```python
from build123d import *

# Parameters (mm, degrees)
SKETCH_1_W                       = 145
SKETCH_1_H                       = 80
EXTRUDE_1_DEPTH                  = 35
SKETCH_2_W                       = 141
SKETCH_2_H                       = 76
CUT_EXTRUDE_1_DEPTH              = 33
SKETCH_3_R                       = 3.5
EXTRUDE_2_DEPTH                  = 15
SKETCH_4_R                       = 1.5
CUT_EXTRUDE_2_DEPTH              = 15
SKETCH_5_W                       = 10
SKETCH_5_H                       = 10
SKETCH_5_W_2                     = 16
SKETCH_5_H_2                     = 21
CUT_EXTRUDE_3_DEPTH              = 15
SKETCH_6_W                       = 10
SKETCH_6_H                       = 10
CUT_EXTRUDE_4_DEPTH              = 15
SKETCH_9_R                       = 3.5
EXTRUDE_3_DEPTH                  = 33
SKETCH_10_R                      = 1.5
CUT_EXTRUDE_5_DEPTH              = 33
PATTERN_LINEAR_2_COUNT           = 2
PATTERN_LINEAR_2_PITCH           = 72
PATTERN_LINEAR_2_COUNT_DIR2      = 2
PATTERN_LINEAR_2_PITCH_DIR2      = 137
SKETCH_12_W                      = 2
SKETCH_12_H                      = 6
EXTRUDE_4_DEPTH                  = 5
SKETCH_13_R                      = 1.5
CUT_EXTRUDE_6_DEPTH              = 5
PATTERN_LINEAR_3_COUNT           = 2
PATTERN_LINEAR_3_PITCH           = 74
PATTERN_LINEAR_4_COUNT           = 2
PATTERN_LINEAR_4_PITCH           = 150
PATTERN_LINEAR_4_COPY_1_SKETCH_R = 1.5
PATTERN_LINEAR_4_COPY_1_DEPTH    = 5


with BuildPart() as part:
    # Эскиз1 → Бобышка-Вытянуть1 (new body)
    with BuildSketch(Plane.XY):
        with Locations((72.5, 40)):
            Rectangle(SKETCH_1_W, SKETCH_1_H)
    extrude(amount=EXTRUDE_1_DEPTH)

    # Эскиз2 → Вырез-Вытянуть1 (cut)
    with BuildSketch(Plane(origin=(0, 0, 0), x_dir=(-1, 0, 0), z_dir=(0, 0, -1))):
        with Locations((-72.5, 40)):
            Rectangle(SKETCH_2_W, SKETCH_2_H)
    extrude(amount=-CUT_EXTRUDE_1_DEPTH, mode=Mode.SUBTRACT)

    # Эскиз3 → Бобышка-Вытянуть2 (add)
    with BuildSketch(Plane(origin=(0, 0, 33), x_dir=(-1, 0, 0), z_dir=(0, 0, -1))):
        with Locations(Location((-109.79, 62.86, 0), (0, 0, 180))):
            Circle(SKETCH_3_R)
        with Locations(Location((-109.79, 17.14, 0), (0, 0, 180))):
            Circle(SKETCH_3_R)
        with Locations(Location((-34.79, 64.13, 0), (0, 0, 180))):
            Circle(SKETCH_3_R)
        with Locations(Location((-34.79, 15.87, 0), (0, 0, 180))):
            Circle(SKETCH_3_R)
    extrude(amount=EXTRUDE_2_DEPTH)

    # Эскиз4 → Вырез-Вытянуть2 (cut)
    with BuildSketch(Plane(origin=(0, 0, 18), x_dir=(-1, 0, 0), z_dir=(0, 0, -1))):
        with Locations((-109.79, 62.86)):
            Circle(SKETCH_4_R)
        with Locations((-34.79, 64.13)):
            Circle(SKETCH_4_R)
        with Locations((-34.79, 15.87)):
            Circle(SKETCH_4_R)
        with Locations((-109.79, 17.14)):
            Circle(SKETCH_4_R)
    extrude(amount=-CUT_EXTRUDE_2_DEPTH, mode=Mode.SUBTRACT)

    # Эскиз5 → Вырез-Вытянуть3 (cut)
    with BuildSketch(Plane.ZY):
        with Locations((13, 26)):
            Rectangle(SKETCH_5_W, SKETCH_5_H)
        with Locations((14, 51.5)):
            Rectangle(SKETCH_5_W_2, SKETCH_5_H_2)
    extrude(amount=-CUT_EXTRUDE_3_DEPTH, mode=Mode.SUBTRACT)

    # Эскиз6 → Вырез-Вытянуть4 (cut)
    with BuildSketch(Plane.ZY.offset(-143)):
        with Locations((13, 54)):
            Rectangle(SKETCH_6_W, SKETCH_6_H)
    extrude(amount=-CUT_EXTRUDE_4_DEPTH, mode=Mode.SUBTRACT)

    # Эскиз9 → Бобышка-Вытянуть3 (add)
    with BuildSketch(Plane(origin=(0, 0, 33), x_dir=(-1, 0, 0), z_dir=(0, 0, -1))):
        with Locations((-4, 76)):
            Circle(SKETCH_9_R)
    extrude_3 = extrude(amount=EXTRUDE_3_DEPTH)

    # Эскиз10 → Вырез-Вытянуть5 (cut)
    with BuildSketch(Plane(origin=(0, 0, 0), x_dir=(-1, 0, 0), z_dir=(0, 0, -1))):
        with Locations((-4, 76)):
            Circle(SKETCH_10_R)
    cut_extrude_5 = extrude(amount=-CUT_EXTRUDE_5_DEPTH, mode=Mode.SUBTRACT)

    # Линейный массив2: Бобышка-Вытянуть3, Cut-Extrude 5 2 × 2
    with Locations(*[(j * PATTERN_LINEAR_2_PITCH_DIR2, -i * PATTERN_LINEAR_2_PITCH, 0) for i in range(PATTERN_LINEAR_2_COUNT) for j in range(PATTERN_LINEAR_2_COUNT_DIR2) if (i, j) != (0, 0)]):
        add(extrude_3)
        add(cut_extrude_5, mode=Mode.SUBTRACT)

    # Эскиз12 → Бобышка-Вытянуть4 (add)
    with BuildSketch(Plane(origin=(145, 0, 0), x_dir=(0, 0, -1), z_dir=(1, 0, 0))):
        with Locations((-34, 77)):
            Rectangle(SKETCH_12_W, SKETCH_12_H)
        with Locations((-34, 3)):
            Rectangle(SKETCH_12_W, SKETCH_12_H)
    extrude_4 = extrude(amount=EXTRUDE_4_DEPTH)

    # Эскиз13 → Вырез-Вытянуть6 (cut)
    with BuildSketch(Plane(origin=(0, 0, 33), x_dir=(-1, 0, 0), z_dir=(0, 0, -1))):
        with Locations((-147.5, 77)):
            Circle(SKETCH_13_R)
    cut_extrude_6 = extrude(amount=-CUT_EXTRUDE_6_DEPTH, mode=Mode.SUBTRACT)

    # Линейный массив3: Вырез-Вытянуть6 ×2
    with Locations(*[(0, -i * PATTERN_LINEAR_3_PITCH, 0) for i in range(1, PATTERN_LINEAR_3_COUNT)]):
        add(cut_extrude_6, mode=Mode.SUBTRACT)

    # Линейный массив4: Бобышка-Вытянуть4, Вырез-Вытянуть6 ×2
    with Locations(*[(-i * PATTERN_LINEAR_4_PITCH, 0, 0) for i in range(1, PATTERN_LINEAR_4_COUNT)]):
        add(extrude_4)
        add(cut_extrude_6, mode=Mode.SUBTRACT)

    # Линейный массив4 copy 1 sketch → Линейный массив4 copy 1 (cut)
    with BuildSketch(Plane(origin=(-150, -74, 33), x_dir=(-1, 0, 0), z_dir=(0, 0, -1))):
        with Locations((-147.5, 77)):
            Circle(PATTERN_LINEAR_4_COPY_1_SKETCH_R)
    extrude(amount=-PATTERN_LINEAR_4_COPY_1_DEPTH, mode=Mode.SUBTRACT)


solid = part.part
```
The model under review builds one solid part; all positions refer to its coordinate system, in mm. A direction names the side the tool comes from. Round coordinates to 2 decimals unless told otherwise and drop trailing zeros. Order: outer loops, then holes, each group sorted by start corner. A loop starts at its lowest first (then second) coordinate and runs counter-clockwise, first axis right, second up. Notation, with made-up numbers: M -36,-3.75 L 17,-3.75 A15 ccw 17,25.25 Z; hole C 13.25,1 d6. An arc over 180 degrees is marked long. Use a Markdown table: item, result.
1) Draft analysis for pull direction X (two halves, no side actions). For faces 4 (the face through (31.293, 15.716, 25.605)), 5 (the face through (71, 80, 18)), state which applies: released by +X, released by -X, zero draft, split by the parting line, or undercut.
Report:
| item | result |
|---|---|
| face 4 | undercut |
| face 5 | zero draft |
2) Consider section B-B (z = 30). Give the number of separate pieces and of enclosed holes in the cut face, then the cut area to 3 significant figures.
Report:
| item | result |
|---|---|
| separate pieces | 5 |
| enclosed holes | 9 |
| area | 1,090 mm^2 |
3) Consider section D-D (x = 147.5). Write out the cut boundary in (y, z).
Report:
| item | result |
|---|---|
| outline | M 0,33 L 1.5,33 L 1.5,35 L 0,35 Z; M 4.5,33 L 6,33 L 6,35 L 4.5,35 Z; M 74,33 L 75.5,33 L 75.5,35 L 74,35 Z; M 78.5,33 L 80,33 L 80,35 L 78.5,35 Z |
4) Consider section A-A (z = 10). Write out the cut boundary in (x, y).
Report:
| item | result |
|---|---|
| outline | M 0,0 L 145,0 L 145,49 L 143,49 L 143,6.87 A3.5 ccw 138.13,2 L 6.87,2 A3.5 ccw 2,6.87 L 2,21 L 0,21 Z; M 0,31 L 2,31 L 2,41 L 0,41 Z; M 0,62 L 2,62 L 2,73.13 A3.5 ccw 6.87,78 L 138.13,78 A3.5 ccw 143,73.13 L 143,59 L 145,59 L 145,80 L 0,80 Z; hole C 4,4 d3; hole C 4,76 d3; hole C 141,4 d3; hole C 141,76 d3 |
5) Wall thickness on line 1 along Y through (x, z) = (-2.5, 33.7); line 2 along Y through (x, z) = (109.79, 29.5); line 3 along X through (y, z) = (77, 34.6): over which ranges is each line inside the solid? List them lowest first. Write a range as [from, to].
Report:
| item | result |
|---|---|
| line 1 | [0, 1.5], [4.5, 6], [74, 75.5], [78.5, 80] |
| line 2 | [0, 2], [13.64, 15.64], [18.64, 20.64], [59.36, 61.36], [64.36, 66.36], [78, 80] |
| line 3 | [-5, -4], [-1, 146], [149, 150] |
6) Insertion check: pin 1 (10 mm diameter, centred on y = 54.5, z = 15, fed in from -X); pin 2 (1.5 mm diameter, centred on x = 141.5, y = 4.5, fed in from -Z); pin 3 (5 mm diameter, centred on y = 41.5, z = 14, fed in from -X). Each pin has a flat end and moves straight along its axis. Give the tip position at first contact, or say it passes through.
Report:
| item | result |
|---|---|
| pin 1 | x = 143 |
| pin 2 | z = 33 |
| pin 3 | x = 0 |
7) Consider section C-C (x = 68). Write out the cut boundary in (y, z), then the cut area to 3 significant figures.
Report:
| item | result |
|---|---|
| outline | M 0,0 L 2,0 L 2,33 L 78,33 L 78,0 L 80,0 L 80,35 L 0,35 Z |
| area | 292 mm^2 |
8) Tool access review of faces 1 (the face through (4, 76, 33)), 2 (the face through (-4.2, 3, 33)), 3 (the face through (-2.175, 1.536, 33.986)): name each direction out of +Z, -Z, +X, -X, +Y, -Y from which nothing blocks a thin tool from reaching the whole face with its end or side.
Report:
| item | result |
|---|---|
| face 1 | -Z |
| face 2 | -Z, -X, +Y, -Y |
| face 3 | +Z, -Z |
